The model under review builds one solid part; all positions refer to its coordinate system, in mm. A direction names the side the tool comes from. Give positions to 0.01 mm unless a question says otherwise; leave off trailing zeros. Loops run counter-clockwise (first coordinate to the right, second up) from the corner with the lowest first, then second, coordinate; pieces in that order, holes last. Notation, with made-up numbers: M 67,7 L 98,7 A20 cw 98,33 Z; hole C 4.5,52 d5. An arc over 180 degrees is marked long. Write item = value, one per line. Start each with the question number.
1. Draft analysis for pull direction X (two halves, no side actions). For faces 1 (the face through (1, 1, 0)), 2 (the face through (18.25, -18.73, -9.57)), 3 (the face through (0, 6.8, 23)), 4 (the face through (-1, 1, 0)), state which applies: pulls with the +X half, pulls with the -X half, needs draft (parallel to the pull), parting line crosses it, or undercut.
2. Wall thickness on line 1 along Z through (x, y) = (3, 12.5); line 2 along X through (y, z) = (-18, -9); line 3 along Y through (x, z) = (24, 11.5) (3 decimals): over which ranges is each line inside the solid? List them lowest first. Write a range as from..to.
3. For faces 5 (the face through (26.14, 11.74, -21.9)), 6 (the face through (-0.01, -3.29, 4.93)), 7 (the face through (15, 10.755, -25)), 8 (the face through (0, -10.245, -23)), list the 3-axis set-ups (+Z, -Z, +X, -X, +Y, -Y) from which the entire face can be reached by the end or side of a thin tool; tool diameter is ignored.
4. We need section A-A on y = 4. Give the boundary of the cut face in (x, z), then the cut area to 3 significant figures.
5. For pin 1 (12 mm diameter, centred on x = 6, y = -15.5, fed in from -Z); pin 2 (4.5 mm diameter, centred on x = 11, y = -17.5, fed in from +Z); pin 3 (10.5 mm diameter, centred on y = -3.745, z = 10.5, fed in from +X); pin 4 (2.5 mm diameter, centred on x = 19.75, z = -9.5, fed in from -Y), all flat-tipped, find the tip position at first contact; note any pin that passes through.
6. We need section B-B on x = 9.5. Give the boundary of the cut face in (y, z) (3 decimals).
from build123d import *

# Parameters (mm, degrees)
BOSS_EXTRUDE1_DEPTH            = 1
CONVERT_SOLID1_START           = -1
CONVERT_SOLID1_DEPTH           = 1
EDGE_FLANGE1_STRIP_W           = 12
EDGE_FLANGE1_STRIP_H           = 2
EDGE_FLANGE1_STRIP_CUT_DEPTH   = 38
EDGE_FLANGE1_DEPTH             = 38
EDGE_FLANGE2_STRIP_W           = 12
EDGE_FLANGE2_STRIP_H           = 2
EDGE_FLANGE2_STRIP_CUT_DEPTH   = 8
EDGE_FLANGE2_STRIP_2_W         = 12
EDGE_FLANGE2_STRIP_2_H         = 2
EDGE_FLANGE2_STRIP_CUT_2_DEPTH = 8
EDGE_FLANGE2_DEPTH             = 8
EDGE_FLANGE2_BEND_DEPTH        = 8
FILLET1_R                      = 3
M3X0_5_TAPPED_HOLE1_D          = 3
SKETCH20_R                     = 4
CUT_EXTRUDE1_DEPTH             = 44.667665669
M4X0_7_TAPPED_HOLE1_D          = 4
M4X0_7_TAPPED_HOLE2_D          = 4
M3X0_5_TAPPED_HOLE2_D          = 3
FILLET2_R                      = 0.2


# Read off the part's stored shape, not the designer's step: Convert-Solid1
# Sheet-metal steps are written as plain solids
with BuildPart() as part:
    # Sketch1 → Boss-Extrude1 (new body)
    with BuildSketch(Plane(origin=(0, 0, 0), x_dir=(0, 0, -1), z_dir=(1, 0, 0))):
        with BuildLine():
            Line((-19, -17.745), (19, -17.745))
            Line((19, -17.745), (19, -10.245))
            Line((19, -10.245), (26, -10.245))
            ThreePointArc((26, -10.245), (28.121320344, -9.366320344), (29, -7.245))
            Line((29, -7.245), (29, 10.755))
            Line((29, 10.755), (21, 10.755))
            Line((21, 10.755), (21, 5.755))
            Line((21, 5.755), (19, 5.755))
            Line((19, 5.755), (19, 14.745))
            ThreePointArc((19, 14.745), (18.121320344, 16.866320344), (16, 17.745))
            Line((16, 17.745), (-16, 17.745))
            ThreePointArc((-16, 17.745), (-18.121320344, 16.866320344), (-19, 14.745))
            Line((-19, 14.745), (-19, 5.755))
            Line((-19, 5.755), (-21, 5.755))
            Line((-21, 5.755), (-21, 10.755))
            Line((-21, 10.755), (-29, 10.755))
            Line((-29, 10.755), (-29, -7.245))
            ThreePointArc((-29, -7.245), (-28.121320344, -9.366320344), (-26, -10.245))
            Line((-26, -10.245), (-19, -10.245))
            Line((-19, -10.245), (-19, -17.745))
        make_face()
    extrude(amount=BOSS_EXTRUDE1_DEPTH)

    # Convert-Solid1 outline → Convert-Solid1 (add)
    with BuildSketch(Plane.YZ.offset(CONVERT_SOLID1_START)):
        with BuildLine():
            Line((17.745, -16), (17.745, 16))
            ThreePointArc((17.745, 16), (16.866320344, 18.121320344), (14.745, 19))
            Line((14.745, 19), (5.755, 19))
            Line((5.755, 19), (5.755, 21))
            Line((5.755, 21), (10.755, 21))
            Line((10.755, 21), (10.755, 29))
            Line((10.755, 29), (-7.245, 29))
            ThreePointArc((-7.245, 29), (-9.366320344, 28.121320344), (-10.245, 26))
            Line((-10.245, 26), (-10.245, 19))
            Line((-10.245, 19), (-17.745, 19))
            Line((-17.745, 19), (-17.745, -19))
            Line((-17.745, -19), (-10.245, -19))
            Line((-10.245, -19), (-10.245, -26))
            ThreePointArc((-10.245, -26), (-9.366320344, -28.121320344), (-7.245, -29))
            Line((-7.245, -29), (10.755, -29))
            Line((10.755, -29), (10.755, -21))
            Line((10.755, -21), (5.755, -21))
            Line((5.755, -21), (5.755, -19))
            Line((5.755, -19), (14.745, -19))
            ThreePointArc((14.745, -19), (16.866320344, -18.121320344), (17.745, -16))
        make_face()
    extrude(amount=CONVERT_SOLID1_DEPTH)

    # Edge-Flange1 strip (across the edge) → Edge-Flange1 strip cut (cut)
    with BuildSketch(Plane(origin=(1, -17.745, 19), x_dir=(0, 1, 0), z_dir=(0, 0, -1))):
        with Locations((-4, -1)):
            Rectangle(EDGE_FLANGE1_STRIP_W, EDGE_FLANGE1_STRIP_H)
    extrude(amount=EDGE_FLANGE1_STRIP_CUT_DEPTH, mode=Mode.SUBTRACT)

    # Edge-Flange1 section (across the edge) → Edge-Flange1 (add)
    with BuildSketch(Plane(origin=(1, -17.745, 19), x_dir=(0, 1, 0), z_dir=(0, 0, -1))):
        with BuildLine():
            Line((-2, 2), (-2, 26))
            Line((-2, 26), (0, 26))
            Line((0, 26), (0, 2))
            ThreePointArc((0, 2), (0.585786438, 0.585786438), (2, 0))
            Line((2, 0), (2, -2))
            ThreePointArc((2, -2), (-0.828427125, -0.828427125), (-2, 2))
        make_face()
    extrude(amount=EDGE_FLANGE1_DEPTH)

    # Edge-Flange2 strip (across the edge) → Edge-Flange2 strip cut (cut)
    with BuildSketch(Plane(origin=(1, 10.755, 21), x_dir=(0, -1, 0), z_dir=(0, 0, 1))):
        with Locations((-4, -1)):
            Rectangle(EDGE_FLANGE2_STRIP_W, EDGE_FLANGE2_STRIP_H)
    extrude(amount=EDGE_FLANGE2_STRIP_CUT_DEPTH, mode=Mode.SUBTRACT)

    # Edge-Flange2 strip 2 (across the edge) → Edge-Flange2 strip cut 2 (cut)
    with BuildSketch(Plane(origin=(1, 10.755, -29), x_dir=(0, -1, 0), z_dir=(0, 0, 1))):
        with Locations((-4, -1)):
            Rectangle(EDGE_FLANGE2_STRIP_2_W, EDGE_FLANGE2_STRIP_2_H)
    extrude(amount=EDGE_FLANGE2_STRIP_CUT_2_DEPTH, mode=Mode.SUBTRACT)

    # Edge-Flange2 section (across the edge) → Edge-Flange2 (add)
    with BuildSketch(Plane(origin=(1, 10.755, 21), x_dir=(0, -1, 0), z_dir=(0, 0, 1))):
        with BuildLine():
            Line((-2, 2), (-2, 26))
            Line((-2, 26), (0, 26))
            Line((0, 26), (0, 2))
            ThreePointArc((0, 2), (0.585786438, 0.585786438), (2, 0))
            Line((2, 0), (2, -2))
            ThreePointArc((2, -2), (-0.828427125, -0.828427125), (-2, 2))
        make_face()
    extrude(amount=EDGE_FLANGE2_DEPTH)

    # Edge-Flange2 section 2 (across the edge) → Edge-Flange2 bend (add)
    with BuildSketch(Plane(origin=(1, 10.755, -29), x_dir=(0, -1, 0), z_dir=(0, 0, 1))):
        with BuildLine():
            Line((-2, 2), (-2, 26))
            Line((-2, 26), (0, 26))
            Line((0, 26), (0, 2))
            ThreePointArc((0, 2), (0.585786438, 0.585786438), (2, 0))
            Line((2, 0), (2, -2))
            ThreePointArc((2, -2), (-0.828427125, -0.828427125), (-2, 2))
        make_face()
    extrude(amount=EDGE_FLANGE2_BEND_DEPTH)

    # Fillet1
    fillet1_edges = [part.edges().sort_by_distance(p)[0] for p in [
        (27, 11.755, 21),
        (27, 11.755, 29),
        (27, 11.755, -29),
        (27, 11.755, -21),
        (27, -18.745, 19),
        (27, -18.745, -19),
    ]]
    fillet(fillet1_edges, radius=FILLET1_R)

    # M3x0.5 Tapped Hole1 (through all)
    with Locations(Plane(origin=(0, -19.745, 0), x_dir=(-1, 0, 0), z_dir=(0, -1, 0))):
        with Locations((-19.75, -9.5), (-7.25, -9.5), (-13.5, -9.5), (-13.5, -3.25), (-13.5, -15.75), (-7.25, 9.5), (-13.5, 3.25), (-19.75, 9.5), (-13.5, 9.5), (-13.5, 15.75)):
            Hole(M3X0_5_TAPPED_HOLE1_D / 2)

    # Sketch20 → Cut-Extrude1 (cut, through all)
    with BuildSketch(Plane(origin=(1, 0, 0), x_dir=(0, 0, -1), z_dir=(1, 0, 0))):
        with Locations((10.5, -3.745)):
            Circle(SKETCH20_R)
        with Locations((0, 6.255)):
            Circle(SKETCH20_R)
        with Locations((-10.5, -3.745)):
            Circle(SKETCH20_R)
    extrude(amount=-CUT_EXTRUDE1_DEPTH, mode=Mode.SUBTRACT)

    # M4x0.7 Tapped Hole1 (through all)
    with Locations(Plane(origin=(0, 10.755, 0), x_dir=(-1, 0, 0), z_dir=(0, -1, 0))):
        with Locations((-18.5, -25), (-8.5, -25), (-8.5, 25), (-18.5, 25)):
            Hole(M4X0_7_TAPPED_HOLE1_D / 2)

    # M4x0.7 Tapped Hole2 (through all)
    with Locations(Plane(origin=(1, 0, 0), x_dir=(0, 0, -1), z_dir=(1, 0, 0))):
        with Locations((25, -3.245), (25, 6.755), (-25, 6.755), (-25, -3.245)):
            Hole(M4X0_7_TAPPED_HOLE2_D / 2)

    # M3x0.5 Tapped Hole2 (through all)
    with Locations(Plane(origin=(1, 0, 0), x_dir=(0, 0, -1), z_dir=(1, 0, 0))):
        with Locations((-10.5, 3.255), (-10.5, -10.745), (-3.5, -3.745), (-17.5, -3.745), (0, 13.255), (0, -0.745), (7, 6.255), (-7, 6.255), (10.5, 3.255), (10.5, -10.745), (17.5, -3.745), (3.5, -3.745)):
            Hole(M3X0_5_TAPPED_HOLE2_D / 2)

    # Fillet2
    fillet2_edges = [part.edges().sort_by_distance(p)[0] for p in [
        (0, 5.755, -19),
        (0, 5.755, -21),
        (0, -10.245, -19),
        (0, -10.245, 19),
        (0, 5.755, 21),
        (0, 5.755, 19),
    ]]
    fillet(fillet2_edges, radius=FILLET2_R)


solid = part.part
Final values:
q1.face_1 = pulls with the +X half
q1.face_2 = undercut
q1.face_3 = needs draft
q1.face_4 = pulls with the -X half
q2.line_1 = -29..-21, 21..29
q2.line_2 = -0.3..5.84, 8.66..12.09, 14.91..18.34, 21.16..27
q2.line_3 = -19.745..-17.745
q3.face_5 = +X, +Y, -Y
q3.face_6 = +X, -X
q3.face_7 = +Z, -Z, +X, -Y
q3.face_8 = -Z, +X, -X, -Y
q4.outline = M -1,-29 L 1,-29 L 1,-11.8 L -1,-11.8 Z; M -1,-9.2 L 1,-9.2 L 1,-3.3 L -1,-3.3 Z; M -1,3.3 L 1,3.3 L 1,9.2 L -1,9.2 Z; M -1,11.8 L 1,11.8 L 1,29 L -1,29 Z
q4.area = 92.4 mm²
q5.pin_1 = -19
q5.pin_2 = 19
q5.pin_3 = 1
q5.pin_4 = through
q6.outline = M -19.745,-19 L -17.745,-19 L -17.745,19 L -19.745,19 Z; M 10.755,-29 L 12.755,-29 L 12.755,-26.732 L 10.755,-26.732 Z; M 10.755,-23.268 L 12.755,-23.268 L 12.755,-21 L 10.755,-21 Z; M 10.755,21 L 12.755,21 L 12.755,23.268 L 10.755,23.268 Z; M 10.755,26.732 L 12.755,26.732 L 12.755,29 L 10.755,29 Z
